Check sheet for the modelled part. Datum: model origin and axes. Units: mm. Face numbers are marked on the shaded views. Give positions to 0.01 mm unless a question says otherwise; leave off trailing zeros. Write each loop counter-clockwise with the first axis right and the second up, starting at its lowest first coordinate (ties: lowest second). Pieces come first, ordered by that corner, then holes. Notation, with made-up numbers: (44, 28) -> (97, 28) arc R20 ccw to (97, 48) -> close; hole circle Ø10 at (76.25, 8.25). An arc over 180 degrees is marked (long way). Use a Markdown table: item, result. Add a question column.
1. Gauge pin test, flat ends, axial feed: P1, Ø1, axis at x = -32.5, y = -17.5, coming from the -Z side; P2, Ø6.5, axis at x = 37, y = 0, coming from the +Z side. Record the tip position at first contact, or that the pin passes through.
2. Cross-section at B-B (y = -30.5). Enter the section's corners in (x, z) (3 decimals).
3. Release check for a two-part mould opening along Y. For the marked faces 1 and 2 record: released by +Y, released by -Y, zero draft, split by the parting line, or undercut.
4. Cross-section at C-C (z = 2.05). Enter the section's corners in (x, y), then the cut area to 3 significant figures.
5. Scan lines: probe 1 along Y at (x, z) = (-19, 2.3); probe 2 along Y at (x, z) = (-18.5, 0.4); probe 3 along Y at (x, z) = (0, 2.75). Record each from-to range of solid material in increasing order. Write a range as [from, to].
from build123d import *

# Parameters (mm, degrees)
SKETCH2_R           = 42.9895
SKETCH2_R_2         = 4.1021
SKETCH2_R_3         = 15.24
BOSS_EXTRUDE2_DEPTH = 3.175
SKETCH3_R           = 31.75
CUT_EXTRUDE1_DEPTH  = 2.38125
CUT_EXTRUDE2_DEPTH  = 4.1275


with BuildPart() as part:
    # Sketch2 → Boss-Extrude2 (new body)
    with BuildSketch(Plane.XY):
        with Locations((-4e-09, 0)):
            Circle(SKETCH2_R)
        with Locations((-18.49755, 32.038696425)):
            Circle(SKETCH2_R_2, mode=Mode.SUBTRACT)
        with Locations((18.49755, 32.038696425)):
            Circle(SKETCH2_R_2, mode=Mode.SUBTRACT)
        with Locations((36.9951, 0)):
            Circle(SKETCH2_R_2, mode=Mode.SUBTRACT)
        with Locations((18.49755, -32.038696425)):
            Circle(SKETCH2_R_2, mode=Mode.SUBTRACT)
        with Locations((-18.49755, -32.038696425)):
            Circle(SKETCH2_R_2, mode=Mode.SUBTRACT)
        with Locations((-36.9951, 0)):
            Circle(SKETCH2_R_2, mode=Mode.SUBTRACT)
        with Locations((-4e-09, 0)):
            Circle(SKETCH2_R_3, mode=Mode.SUBTRACT)
    extrude(amount=BOSS_EXTRUDE2_DEPTH)

    # Sketch3 → Cut-Extrude1 (cut)
    with BuildSketch(Plane.XY.offset(3.175)):
        with Locations((-4e-09, 0)):
            Circle(SKETCH3_R)
    extrude(amount=-CUT_EXTRUDE1_DEPTH, mode=Mode.SUBTRACT)

    # Sketch3<3> → Cut-Extrude2 (cut)
    with BuildSketch(Plane.XY.offset(3.175)):
        Polygon((-7.185170954, 13.439900239), (37.844396615, 37.513378093), (51.563249181, 10.3209669), (6.307069446, -13.873661195), align=None)
    extrude(amount=-CUT_EXTRUDE2_DEPTH, mode=Mode.SUBTRACT)


solid = part.part
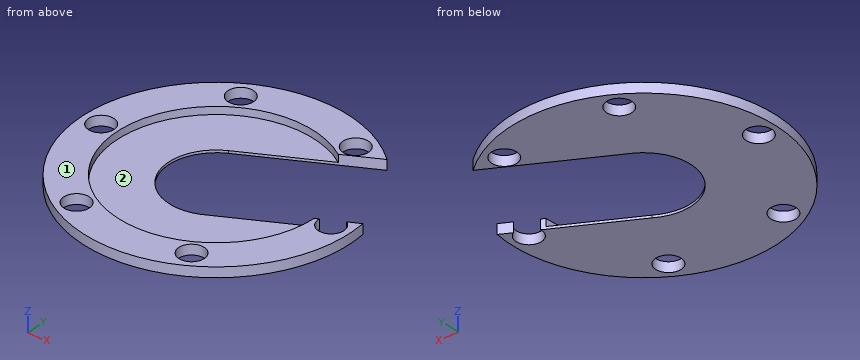
Worked answers:
| question | item | result |
|---|---|---|
| 1 | P1 | stops at z = 0 |
| 1 | P2 | passes through |
| 2 | outline | (-30.296, 0) -> (-22.3, 0) -> (-22.3, 3.175) -> (-30.296, 3.175) -> close; (-14.695, 0) -> (14.695, 0) -> (14.695, 3.175) -> (8.821, 3.175) -> (8.821, 0.794) -> (-8.821, 0.794) -> (-8.821, 3.175) -> (-14.695, 3.175) -> close; (22.3, 0) -> (30.296, 0) -> (30.296, 3.175) -> (22.3, 3.175) -> close |
| 3 | face 1 | zero draft |
| 3 | face 2 | undercut |
| 4 | outline | (17.38, 26.57) -> (28.26, 32.39) arc R42.99 ccw (long way) to (42.63, 5.55) -> (38.98, 3.59) arc R4.1 cw (long way) to (32.91, 0.35) -> (31.75, -0.27) arc R31.75 cw (long way) to start; hole circle Ø8.2 at (-37, 0); hole circle Ø8.2 at (-18.5, -32.04); hole circle Ø8.2 at (-18.5, 32.04); hole circle Ø8.2 at (18.5, -32.04); hole circle Ø8.2 at (18.5, 32.04) |
| 4 | area | 1,980 mm² |
| 5 | probe 1 | y = [-38.56, -36.11], [-27.97, -25.44], [25.44, 27.97], [36.11, 38.56] |
| 5 | probe 2 | y = [-38.81, -36.14], [-27.94, 27.94], [36.14, 38.81] |
| 5 | probe 3 | y = [-42.99, -31.75], [31.75, 42.99] |
